```python
from build123d import *

# Parameters (mm, degrees)
BOSS_EXTRU_1_DEPTH      = 3
ENL_V_MAT_EXTRU_1_DEPTH = 345.268848431
ESQUISSE3_R             = 1.5
ENL_V_MAT_EXTRU_2_DEPTH = 331.898715622
ESQUISSE4_R             = 8
ENL_V_MAT_EXTRU_3_DEPTH = 331.898715622
ESQUISSE5_R             = 1.5
ENL_V_MAT_EXTRU_4_DEPTH = 331.898715622


with BuildPart() as part:
    # Esquisse1 → Boss.-Extru.1 (new body)
    with BuildSketch(Plane.XY):
        Polygon((0, 0), (0, 127.45), (65.1, 200), (215.1, 200), (280.2, 127.45), (280.2, 0), align=None)
    extrude(amount=BOSS_EXTRU_1_DEPTH)

    # Esquisse2 → Enlèv. mat.-Extru.1 (cut, through all)
    with BuildSketch(Plane(origin=(0, 0, 0), x_dir=(-1, 0, 0), z_dir=(0, 0, -1))):
        Polygon((-16.6, 0), (-16.6, 145.969439351), (0, 127.45), (0, 0), align=None)
        Polygon((-280.2, 127.45), (-263.6, 145.969439351), (-263.6, 0), (-280.2, 0), align=None)
    extrude(amount=-ENL_V_MAT_EXTRU_1_DEPTH, mode=Mode.SUBTRACT)

    # Esquisse3 → Enlèv. mat.-Extru.2 (cut, through all)
    with BuildSketch(Plane.XY.offset(3)):
        with Locations((78.1, 163.5)):
            Circle(ESQUISSE3_R)
        with Locations((78.1, 36.5)):
            Circle(ESQUISSE3_R)
        with Locations(Location((202.1, 36.5, 0), (0, 0, 180))):
            Circle(ESQUISSE3_R)
        with Locations(Location((202.1, 163.5, 0), (0, 0, 180))):
            Circle(ESQUISSE3_R)
    extrude(amount=-ENL_V_MAT_EXTRU_2_DEPTH, mode=Mode.SUBTRACT)

    # Esquisse4 → Enlèv. mat.-Extru.3 (cut, through all)
    with BuildSketch(Plane.XY.offset(3)):
        with Locations((46.6, 30)):
            Circle(ESQUISSE4_R)
    extrude(amount=-ENL_V_MAT_EXTRU_3_DEPTH, mode=Mode.SUBTRACT)

    # Esquisse5 → Enlèv. mat.-Extru.4 (cut, through all)
    with BuildSketch(Plane.XY.offset(3)):
        with Locations((105.1, 65)):
            Circle(ESQUISSE5_R)
        with Locations((105.1, 135)):
            Circle(ESQUISSE5_R)
        with Locations((175.1, 135)):
            Circle(ESQUISSE5_R)
        with Locations((175.1, 65)):
            Circle(ESQUISSE5_R)
    extrude(amount=-ENL_V_MAT_EXTRU_4_DEPTH, mode=Mode.SUBTRACT)


solid = part.part
```
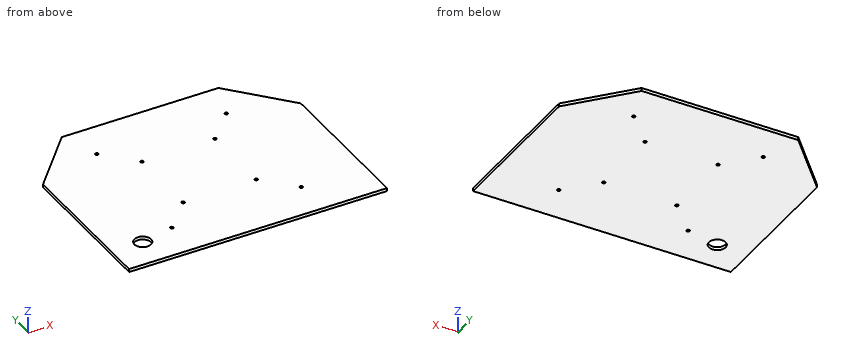
Could you check a few things on this model? Use its own coordinates, in mm. Round coordinates to 2 decimals unless told otherwise and drop trailing zeros. Loops run counter-clockwise (first coordinate to the right, second up) from the corner with the lowest first, then second, coordinate; pieces in that order, holes last. Notation, with made-up numbers: (-16.5, -4) - (15.5, -4) arc R20 ccw to (15.5, 12) - close; hole circle Ø10 at (-14, 38). An arc over 180 degrees is marked (long way). Answer as CSV lines item,"result".
1. For pin 1 Ø3.5 at (x, y) = (175.1, 135) entering from +Z; pin 2 Ø2.5 at (x, y) = (78.1, 36.5) entering from +Z, each with a flat end and sliding along its axis, tell me the tip position at first contact or that it passes through.
Filled in:
pin 1,"stops at z = 3"
pin 2,"passes through"
2. I want a section at B-B on x = 46.6. List the corners of the cut face in (y, z) for me.
Filled in:
outline,"(0, 0) - (22, 0) - (22, 3) - (0, 3) - close; (38, 0) - (179.38, 0) - (179.38, 3) - (38, 3) - close"
3. Please list where these lines run through material, in increasing order: line 1 along Y through (x, z) = (175.1, 2.15); line 2 along X through (y, z) = (65, 1.85); line 3 along Y through (x, z) = (78.1, 1.5). Write a range as [from, to].
Filled in:
line 1,"y = [0, 63.5], [66.5, 133.5], [136.5, 200]"
line 2,"x = [16.6, 103.6], [106.6, 173.6], [176.6, 263.6]"
line 3,"y = [0, 35], [38, 162], [165, 200]"
4. I want a section at D-D on x = 238. List the corners of the cut face in (y, z) for me.
Filled in:
outline,"(0, 0) - (174.48, 0) - (174.48, 3) - (0, 3) - close"
5. I want a section at C-C on y = 157.5. List the corners of the cut face in (x, z) for me.
Filled in:
outline,"(26.96, 0) - (253.24, 0) - (253.24, 3) - (26.96, 3) - close"
6. I want a section at A-A on z = 0.85. Count the separate pieces of the cut face and the enclosed holes in it, then the cut area to 3 significant figures.
Filled in:
separate pieces,"1"
enclosed holes,"9"
area,"46,500 mm^2"
